```python
from build123d import *

# Parameters (mm, degrees)
F1_DEPTH = 1.6
F2_W     = 19
F2_H     = 25
F3_DEPTH = 5.6
F4_W     = 7
F4_H     = 22.1
F5_DEPTH = 8.4
F6_W     = 3
F6_H     = 3
F6_R     = 0.5
F7_DEPTH = 0.75
F8_R     = 1.75
F9_DEPTH = 2


with BuildPart() as f1:
    # F0 (on Top) → F1 (new body)
    with BuildSketch(Plane.XY):
        with BuildLine():
            Line((-22.5, -22.5), (14.5, -22.5))
            Line((14.5, -22.5), (14.5, -16.5))
            ThreePointArc((14.5, -16.5), (15.085786, -15.085786), (16.5, -14.5))
            Line((16.5, -14.5), (22.5, -14.5))
            Line((22.5, -14.5), (22.5, 22.5))
            Line((22.5, 22.5), (-14.5, 22.5))
            Line((-14.5, 22.5), (-14.5, 16.5))
            ThreePointArc((-14.5, 16.5), (-15.085786, 15.085786), (-16.5, 14.5))
            Line((-16.5, 14.5), (-22.5, 14.5))
            Line((-22.5, 14.5), (-22.5, -22.5))
        make_face()
    extrude(amount=F1_DEPTH)

    # F2 (on face) → F3 (join)
    with BuildSketch(Plane.XY.offset(1.6)):
        with Locations((-2.789866, 7.80402)):
            Rectangle(F2_W, F2_H)
    extrude(amount=-F3_DEPTH)

    # F4 (on face) → F5 (join)
    with BuildSketch(Plane.XY.offset(1.6)):
        with Locations((19, 11.45)):
            Rectangle(F4_W, F4_H)
    extrude(amount=F5_DEPTH)

    # F6 (on face) → F7 (join)
    with BuildSketch(Plane.XY.offset(1.6)):
        with Locations((-20, -20)):
            Rectangle(F6_W, F6_H)
        with Locations((-16.867438, -20)):
            Circle(F6_R)
    extrude(amount=F7_DEPTH)

    # F8 (on face) → F9 (cut)
    with BuildSketch(Plane(origin=(0, 0, 0), x_dir=(1, 0, 0), z_dir=(0, 0, -1))):
        with Locations((-18.5, -10.5)):
            Circle(F8_R)
        with Locations((18.5, 10.5)):
            Circle(F8_R)
    extrude(amount=-F9_DEPTH, mode=Mode.SUBTRACT)


solid = f1.part
```
Design review of the part built by this model. Coordinates are the model's own, in mm. A direction names the side the tool comes from. Coordinates: 2 decimals unless noted, no trailing zeros. Loops run counter-clockwise (first coordinate to the right, second up) from the corner with the lowest first, then second, coordinate; pieces in that order, holes last.
Q1. We need section B-B on x = 18.5. State the section outline as (y, z) points, and give its area (3 significant figures).
Reported:
outline: (-14.5, 0) - (-12.25, 0) - (-12.25, 1.6) - (-14.5, 1.6) - close; (-8.75, 0) - (22.5, 0) - (22.5, 10) - (0.4, 10) - (0.4, 1.6) - (-8.75, 1.6) - close
area: 239 mm2
Q2. The part is to be moulded in two halves that separate along Y. For faces 5 (the face through (-19, 14.5, 1)), 6 (the face through (-19.79, 9.32, 0.79)), 7 (the face through (17.21, -11.68, 0.79)), 8 (the face through (-4, -22.5, 1)), say which applies: +Y half, -Y half, draft (parallel to the pull), parting line (faces both ways), or undercut.
Reported:
face 5: +Y half
face 6: undercut
face 7: undercut
face 8: -Y half
Q3. We need section C-C on z = 1. State the section outline as (x, y) points.
Reported:
outline: (-22.5, -22.5) - (14.5, -22.5) - (14.5, -16.5) arc R2 cw to (16.5, -14.5) - (22.5, -14.5) - (22.5, 22.5) - (-14.5, 22.5) - (-14.5, 16.5) arc R2 cw to (-16.5, 14.5) - (-22.5, 14.5) - close; hole circle Ø3.5 at (-18.5, 10.5); hole circle Ø3.5 at (18.5, -10.5)
Q4. We need section A-A on y = 10.5. State the section outline as (x, z) points.
Reported:
outline: (-22.5, 0) - (-20.25, 0) - (-20.25, 1.6) - (-22.5, 1.6) - close; (-16.75, 0) - (-12.29, 0) - (-12.29, -4) - (6.71, -4) - (6.71, 0) - (22.5, 0) - (22.5, 10) - (15.5, 10) - (15.5, 1.6) - (-16.75, 1.6) - close
Q5. For pin 1 (1.3 mm diameter, centred on x = -19, z = 0.5, fed in from +Y); pin 2 (0.6 mm diameter, centred on y = -20, z = 2, fed in from -X); pin 3 (2 mm diameter, centred on y = 9.5, z = -1.5, fed in from +X); pin 4 (2 mm diameter, centred on x = 3, z = 2.5, fed in from -Y), all flat-tipped, find the tip position at first contact; note any pin that passes through.
Reported:
pin 1: stops at y = 14.5
pin 2: stops at x = -21.5
pin 3: stops at x = 6.71
pin 4: stops at y = -22.5
Q6. We need section D-D on y = 1. State the section outline as (x, z) points.
Reported:
outline: (-22.5, 0) - (-12.29, 0) - (-12.29, -4) - (6.71, -4) - (6.71, 0) - (22.5, 0) - (22.5, 10) - (15.5, 10) - (15.5, 1.6) - (-22.5, 1.6) - close
Q7. Tool access review of faces 1 (the face through (14.5, -20, 1)), 2 (the face through (6.71, 8, -2)), 3 (the face through (-3, -4.696, -2)), 4 (the face through (19, 0.4, 6)): name each direction out of +Z, -Z, +X, -X, +Y, -Y from which nothing blocks a thin tool from reaching the whole face with its end or side.
Reported:
face 1: +Z, -Z, +X, -Y
face 2: -Z, +X, +Y, -Y
face 3: -Z, +X, -X, -Y
face 4: +Z, +X, -X, -Y
Q8. To check wall thickness, follow line 1 (X direction, y = 10.5, z = 0.75); line 2 (Y direction, x = -18.5, z = 1.3); line 3 (X direction, y = 8, z = 2.5). State the ranges of each line that lie inside material, in increasing order.
Reported:
line 1: x = -22.5 to -20.25, -16.75 to 22.5
line 2: y = -22.5 to 8.75, 12.25 to 14.5
line 3: x = 15.5 to 22.5
